Answer from the drawing. Dimensions are ordinates in mm from the lowest x, y and z of the part. Coordinates: 2 decimals unless noted, no trailing zeros. Write each loop counter-clockwise with the first axis right and the second up, starting at its lowest first coordinate (ties: lowest second). Pieces come first, ordered by that corner, then holes.
(1) Section A-A on x = 15 is taken. Write down the section's boundary in (y, z), then the cut area to 3 significant figures.
(2) Section B-B on y = 75 is taken. Write down the section's boundary in (x, z), then the cut area to 3 significant figures.
(3) Find the intervals of material crossed by probe 1 along Y at (x, z) = (15, 0.45); probe 2 along X at (y, z) = (15, 0.5); probe 3 along X at (y, z) = (75, 0.75), in increasing order.
(4) Section D-D on z = 1.55 is taken. Write down the section's boundary in (x, y).
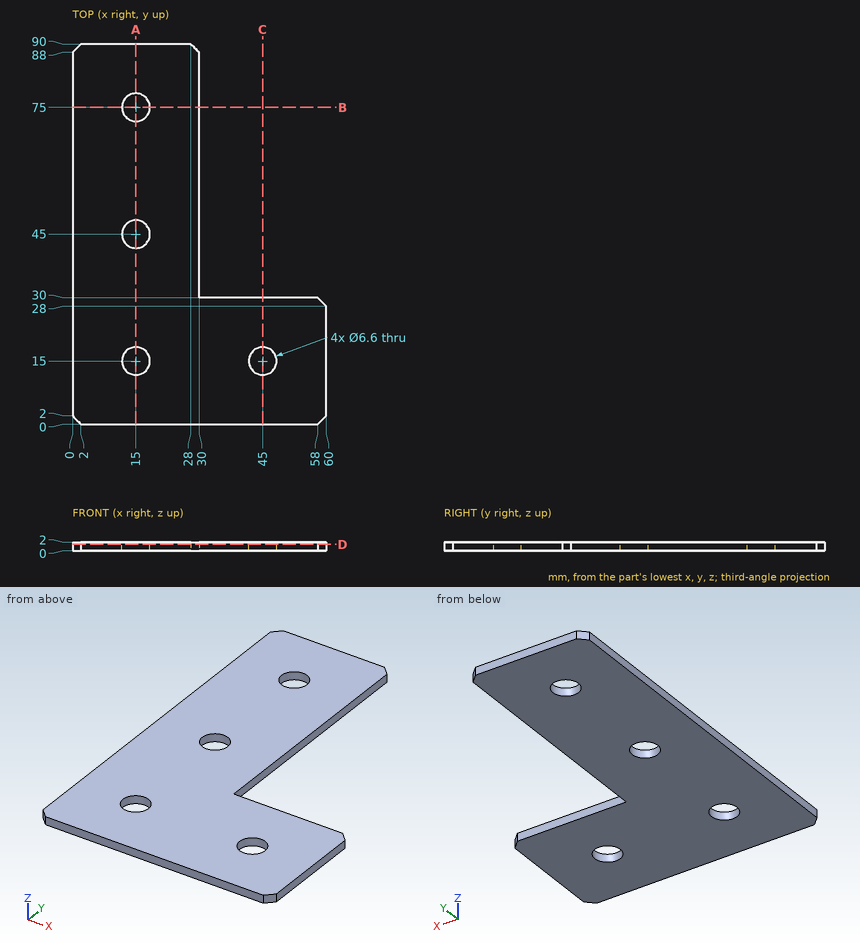
Response:
1. outline: (0, 0) - (11.7, 0) - (11.7, 2) - (0, 2) - close; (18.3, 0) - (41.7, 0) - (41.7, 2) - (18.3, 2) - close; (48.3, 0) - (71.7, 0) - (71.7, 2) - (48.3, 2) - close; (78.3, 0) - (90, 0) - (90, 2) - (78.3, 2) - close
1. area: 140 mm2
2. outline: (0, 0) - (11.7, 0) - (11.7, 2) - (0, 2) - close; (18.3, 0) - (30, 0) - (30, 2) - (18.3, 2) - close
2. area: 46.8 mm2
3. probe 1: y = 0 to 11.7, 18.3 to 41.7, 48.3 to 71.7, 78.3 to 90
3. probe 2: x = 0 to 11.7, 18.3 to 41.7, 48.3 to 60
3. probe 3: x = 0 to 11.7, 18.3 to 30
4. outline: (0, 2) - (2, 0) - (58, 0) - (60, 2) - (60, 28) - (58, 30) - (30, 30) - (30, 88) - (28, 90) - (2, 90) - (0, 88) - close; hole circle Ø6.6 at (15, 15); hole circle Ø6.6 at (15, 45); hole circle Ø6.6 at (15, 75); hole circle Ø6.6 at (45, 15)
